The listing builds one solid part. Answer for the finished solid, in the listing's coordinates (mm). Give positions to 0.01 mm unless a question says otherwise; leave off trailing zeros. Order: outer loops, then holes, each group sorted by start corner. A loop starts at its lowest first (then second) coordinate and runs counter-clockwise, first axis right, second up. Notation, with made-up numbers: (-32, -38.75) - (20, -38.75) arc R19 cw to (20, -26.75) - close; hole circle Ø9 at (12.25, 43). An arc over 180 degrees is marked (long way). Use CSV: the item, a comma, the result in double quotes.
```python
from build123d import *

# Parameters (mm, degrees)
BOSS_EXTRU_1_DEPTH = 10


with BuildPart() as part:
    # Esquisse1 → Boss.-Extru.1 (new body)
    with BuildSketch(Plane.XY):
        with BuildLine():
            Line((0, 20), (0, 50))
            Line((0, 50), (9.138501945, 50))
            ThreePointArc((9.138501945, 50), (19.351259857, 48.20814733), (28.344033934, 43.046638388))
            Line((28.344033934, 43.046638388), (39.20553199, 33.995390008))
            ThreePointArc((39.20553199, 33.995390008), (47.167682637, 23.673413508), (50, 10.94875162))
            Line((50, 10.94875162), (50, 0))
            Line((50, 0), (20, 0))
            Line((20, 0), (0, 20))
        make_face()
    extrude(amount=BOSS_EXTRU_1_DEPTH)


solid = part.part
```
Item 1: The part is cut by section C-C (x = 40). Give the vertices of the cut face in (y, z), and give its area (3 significant figures).
Taken from the geometry:
outline,"(0, 0) - (33.31, 0) - (33.31, 10) - (0, 10) - close"
area,"333 mm^2"
Item 2: This flat-tipped pin is pushed along its axis until it touches: pin 1 (3 mm diameter, centred on y = 40.5, z = 6, fed in from +X). Where does it stop, or does it pass through?
Taken from the geometry:
pin 1,"x = 33.2"
Item 3: The part is cut by section A-A (z = 3.5). Give the vertices of the cut face in (x, y), and give its area (3 significant figures).
Taken from the geometry:
outline,"(0, 20) - (20, 0) - (50, 0) - (50, 10.95) arc R30 ccw to (39.21, 34) - (28.34, 43.05) arc R30 ccw to (9.14, 50) - (0, 50) - close"
area,"1,880 mm^2"
Item 4: Find the intervals of material crossed by line 1 along Y through (x, z) = (45.5, 3.25); line 2 along Y through (x, z) = (36.5, 7.5); line 3 along X through (y, z) = (17.5, 9.5), in increasing order.
Taken from the geometry:
line 1,"0 to 26.75"
line 2,"0 to 36.25"
line 3,"2.5 to 49.28"
Item 5: The part is cut by section B-B (y = 41.5). Give the vertices of the cut face in (x, z), and give its area (3 significant figures).
Taken from the geometry:
outline,"(0, 0) - (30.2, 0) - (30.2, 10) - (0, 10) - close"
area,"302 mm^2"
